Geometry: final body of the model. Coordinates: model frame, mm. A direction names the side the tool comes from. Give positions to 0.01 mm unless a question says otherwise; leave off trailing zeros. Order: outer loops, then holes, each group sorted by start corner. A loop starts at its lowest first (then second) coordinate and runs counter-clockwise, first axis right, second up. Notation, with made-up numbers: M 89.5,56 L 107.5,56 A21 cw 107.5,63 Z; hole C -12.75,64.5 d6. An arc over 180 degrees is marked long. Use CSV: the item, a comma, the result in double quotes.
Autodesk Inventor part; units mm, degrees
ref_plane "YZ Plane" through (0, 0, 0) normal (1, 0, 0) x (0, 1, 0)
ref_plane "XZ Plane" through (0, 0, 0) normal (0, 1, 0) x (-1, 0, 0)
ref_plane "XY Plane" through (0, 0, 0) normal (0, 0, 1) x (1, 0, 0)
sketch "スケッチ1" plane through (0, 0, 0) normal (0, 0, 1) x (1, 0, 0)
  line L0 (10, -10) -> (-10, -10)
  line L1 (-10, -10) -> (-10, 10)
  line L2 (-10, 10) -> (10, 10)
  line L3 (10, 10) -> (10, -10)
  line L4 (10, -10) -> (-10, 10) construction
  line L5 (-10, -10) -> (10, 10) construction
  line L6 (9, 9) -> (-9, 9)
  line L7 (-9, 9) -> (-9, -9)
  line L8 (-9, -9) -> (9, -9)
  line L9 (9, -9) -> (9, 9)
  point P0 (0, 0)
  dimension "d0" = 20
  dimension "d1" = 20
  dimension "d2" = 1
extrude "押し出し1" add sketch "スケッチ1" along normal blind 465
sketch "スケッチ2" plane through (10, -10, 0) normal (1, 0, 0) x (0, 0, -1)
  line L0 (0, 10) -> (-465, 10)
  line L1 (-465, 0) -> (-465, 20)
  line L2 (0, 0) -> (0, 20)
  point P0 (-403, 10)
  point P1 (-60, 10)
  point P2 (-10, 10)
  point P3 (-453, 10)
  point P4 (-82.5, 10)
  point P5 (-232.5, 10)
  dimension "d5" = 343
  dimension "d6" = 50
  dimension "d7" = 10
  dimension "d15" = 50
  dimension "d17" = 465
  dimension "d28" = 150
hole "穴1" at (10, 0, 403) at (10, 0, 60) at (10, 0, 10) at (10, 0, 453) at (10, 0, 82.5) direction (-1, 0, 0) diameter 3.3 end through all
sketch "スケッチ3" plane through (-10, 10, 0) normal (0, 1, 0) x (1, 0, 0)
  line L0 (10, 0) -> (10, -465)
  line L1 (20, -465) -> (0, -465)
  point P0 (10, -242.5)
  point P1 (10, -222.5)
  point P2 (10, -232.5)
  dimension "d19" = 20
  dimension "d20" = 10
hole "穴2" at (0, 10, 242.5) at (0, 10, 222.5) direction (0, -1, 0) diameter 3.3 end through all
sketch "スケッチ6" plane through (0, 0, 0) normal (0, 0, -1) x (-1, 0, 0)
  line L0 (-10, 10) -> (10, 10)
  line L1 (-10, -10) -> (-10, 10)
  line L2 (10, -10) -> (-10, -10)
  line L3 (10, 10) -> (10, -10)
  line L4 (-9, 9) -> (-9, -9)
  line L5 (9, 9) -> (-9, 9)
  line L6 (9, -9) -> (9, 9)
  line L7 (-9, -9) -> (9, -9)
  point P0 (0, 0)
extrude "押し出し4" add sketch "スケッチ6" along normal blind 50
sketch "スケッチ7" plane through (-10, 10, 465) normal (0, 1, 0) x (1, 0, 0)
  line L0 (10, 465) -> (10, 515)
  line L1 (1, 515) -> (19, 515)
  point P0 (10, 500)
  point P1 (10, 485)
  point P2 (10, 495)
  dimension "d44" = 35
  dimension "d52" = 10
  dimension "d53" = 5
hole "穴3" at (0, 10, -30) at (0, 10, -20) at (0, 10, -35) direction (0, -1, 0) diameter 4 end through all
properties part number "kaku_2020_465"
1. Pin query (flat end, axial travel): pin 1 Ø5.5 at (y, z) = (0, 10) entering from +X; pin 2 Ø2.5 at (y, z) = (0, 403) entering from +X. Return the tip coordinate at first contact, or that it passes through.
Answer:
pin 1,"x = 10"
pin 2,"through"
2. Section A-A, the plane x = -5. Return the cut outline in (y, z).
Answer:
outline,"M -10,-50 L -9,-50 L -9,465 L -10,465 Z; M 9,-50 L 10,-50 L 10,465 L 9,465 Z"
3. Section B-B, the plane z = 91.5. Return the cut outline in (x, y).
Answer:
outline,"M -10,-10 L 10,-10 L 10,10 L -10,10 Z; hole M -9,-9 L 9,-9 L 9,9 L -9,9 Z"
4. Pull-direction query (Y, two-part tool) for faces 3 (the face through (0, -9, 211)), 4 (the face through (0, 10, 211)), 5 (the face through (-0.8, -9.6, 465)); classes: +Y half, -Y half, draft (parallel to the pull), parting line (faces both ways), or undercut.
Answer:
face 3,"undercut"
face 4,"+Y half"
face 5,"draft"
5. Reachability of faces 1 (the face through (-10, 0, 211)), 2 (the face through (0, 9, 211)) from +Z, -Z, +X, -X, +Y, -Y: full face, straight path, thin tool, end or side. Return the list, or none.
Answer:
face 1,"+Z, -Z, -X, +Y, -Y"
face 2,"+Z, -Z"
6. Line query: line 1 (Z direction, x = 9.6, y = 0); line 2 (Y direction, x = 9.45, z = 403); line 3 (Y direction, x = 5, z = 137). Output: solid intervals per line, ascending.
Answer:
line 1,"-50 to 8.35, 11.65 to 58.35, 61.65 to 80.85, 84.15 to 401.35, 404.65 to 451.35, 454.65 to 465"
line 2,"-10 to -1.65, 1.65 to 10"
line 3,"-10 to -9, 9 to 10"
